```python
from build123d import *

# Parameters (mm, degrees)
BOSS_EXTRUDE1_DEPTH   = 100
M6_TAPPED_HOLE2_D     = 5
M6_TAPPED_HOLE2_DEPTH = 13.497848452
M6_TAPPED_HOLE2_TIP   = 1.502151548
SKETCH9_R             = 6
CUT_EXTRUDE2_DEPTH    = 2.6
SKETCH10_R            = 2.75
CUT_EXTRUDE3_DEPTH    = 11
SKETCH11_R            = 5.5
CUT_EXTRUDE4_DEPTH    = 5.5


with BuildPart() as part:
    # Sketch1 → Boss-Extrude1 (new body)
    with BuildSketch(Plane(origin=(0, 0, 0), x_dir=(1, 0, 0), z_dir=(0, 1, 0))):
        Polygon((0, 0), (30, 0), (30, 260), (180, 260), (180, 0), (210, 0), (210, 10), (190, 10), (190, 270), (20, 270), (20, 10), (0, 10), align=None)
    extrude(amount=BOSS_EXTRUDE1_DEPTH)

    # M6 Tapped Hole2
    with Locations(Plane(origin=(0, 0, -270), x_dir=(-1, 0, 0), z_dir=(0, 0, -1))):
        with Locations((-145, 50), (-65, 50)):
            Hole(M6_TAPPED_HOLE2_D / 2, depth=M6_TAPPED_HOLE2_DEPTH)
            with Locations((0, 0, -(M6_TAPPED_HOLE2_DEPTH + M6_TAPPED_HOLE2_TIP / 2))):  # 118° drill point
                Cone(0, M6_TAPPED_HOLE2_D / 2, M6_TAPPED_HOLE2_TIP, mode=Mode.SUBTRACT)

    # Sketch9 → Cut-Extrude2 (cut)
    with BuildSketch(Plane(origin=(0, 0, -270), x_dir=(-1, 0, 0), z_dir=(0, 0, -1))):
        with Locations((-145, 50)):
            Circle(SKETCH9_R)
        with Locations((-65, 50)):
            Circle(SKETCH9_R)
    extrude(amount=-CUT_EXTRUDE2_DEPTH, mode=Mode.SUBTRACT)

    # Sketch10 → Cut-Extrude3 (cut, through all)
    with BuildSketch(Plane(origin=(0, 0, -10), x_dir=(-1, 0, 0), z_dir=(0, 0, -1))):
        with Locations((-10, 87.5)):
            Circle(SKETCH10_R)
        with Locations((-10, 12.5)):
            Circle(SKETCH10_R)
        with Locations((-200, 12.5)):
            Circle(SKETCH10_R)
        with Locations((-200, 87.5)):
            Circle(SKETCH10_R)
    extrude(amount=-CUT_EXTRUDE3_DEPTH, mode=Mode.SUBTRACT)

    # Sketch11 → Cut-Extrude4 (cut)
    with BuildSketch(Plane(origin=(0, 0, -10), x_dir=(-1, 0, 0), z_dir=(0, 0, -1))):
        with Locations((-10, 87.5)):
            Circle(SKETCH11_R)
        with Locations((-10, 12.5)):
            Circle(SKETCH11_R)
        with Locations((-200, 12.5)):
            Circle(SKETCH11_R)
        with Locations((-200, 87.5)):
            Circle(SKETCH11_R)
    extrude(amount=-CUT_EXTRUDE4_DEPTH, mode=Mode.SUBTRACT)


solid = part.part
```
Here's how the part is built. I have some questions about the finished solid (model axes, mm). A direction names the side the tool comes from. Give positions to 0.01 mm unless a question says otherwise; leave off trailing zeros. Order: outer loops, then holes, each group sorted by start corner. A loop starts at its lowest first (then second) coordinate and runs counter-clockwise, first axis right, second up. Notation, with made-up numbers: M -30,16.5 L 27,16.5 A21 cw 27,25.5 Z; hole C 48.25,61.5 d11. An arc over 180 degrees is marked long. Use a Markdown table: item, result. Add a question column.
1. For pin 1 Ø5.5 at (x, y) = (9.5, 90) entering from -Z; pin 2 Ø10 at (x, y) = (14.5, 70.5) entering from -Z; pin 3 Ø5 at (y, z) = (23.5, -195.5) entering from -X, each with a flat end and sliding along its axis, tell me the tip position at first contact or that it passes through.
2. I need wall thicknesses on probe 1 along Y at (x, z) = (200, -6); probe 2 along X at (y, z) = (92, -68.5); probe 3 along Z at (x, y) = (49.5, 79). Which ranges of each line are inside material? Lowest first, please. Write a range as from..to.
3. Suppose I cut it at A-A (z = -83.5). List the corners of the cut face in (x, y) for me.
4. If we mould it in two halves opening along X, with no side actions, what happens to faces 1 (the cylindrical face through (7.5, 7.6, -7.3)), 2 (the flat face through (0, 49, -5)), 3 (the flat face through (27, 100, -156))? For each: +X half, -X half, draft (parallel to the pull), parting line (faces both ways), or undercut.
5. Suppose I cut it at B-B (y = 76.5). List the corners of the cut face in (x, z) for me, and give its area (3 significant figures).
6. Suppose I cut it at C-C (x = 88). List the corners of the cut face in (y, z) for me, and give its area (3 significant figures).
7. On a 3-axis mill with a long thin cutter (end or side, diameter ignored), from which of +Z, -Z, +X, -X, +Y, -Y can I reach the whole of each face in a straight line? I mean faces 4 (the flat face through (104, 49, -260)), 5 (the flat face through (106, 49, -270)), 6 (the flat face through (10, 49, -10)), 7 (the flat face through (65, 47, -267.4)). Say none if no direction works.
Results list:
| question | item | result |
|---|---|---|
| 1 | pin 1 | stops at z = -4.5 |
| 1 | pin 2 | stops at z = -10 |
| 1 | pin 3 | stops at x = 20 |
| 2 | probe 1 | y = 0..7, 18..82, 93..100 |
| 2 | probe 2 | x = 20..30, 180..190 |
| 2 | probe 3 | z = -270..-260 |
| 3 | outline | M 20,0 L 30,0 L 30,100 L 20,100 Z; M 180,0 L 190,0 L 190,100 L 180,100 Z |
| 4 | face 1 | undercut |
| 4 | face 2 | -X half |
| 4 | face 3 | draft |
| 5 | outline | M 0,-10 L 20,-10 L 20,-270 L 190,-270 L 190,-10 L 210,-10 L 210,0 L 180,0 L 180,-260 L 30,-260 L 30,0 L 0,0 Z |
| 5 | area | 7,300 mm² |
| 6 | outline | M 0,-270 L 100,-270 L 100,-260 L 0,-260 Z |
| 6 | area | 1,000 mm² |
| 7 | face 4 | +Z, +Y, -Y |
| 7 | face 5 | -Z, +X, -X, +Y, -Y |
| 7 | face 6 | -Z, -X, +Y, -Y |
| 7 | face 7 | -Z |
